Check sheet for the modelled part. Datum: model origin and axes. Units: mm. A direction names the side the tool comes from. Give positions to 0.01 mm unless a question says otherwise; leave off trailing zeros. Write each loop counter-clockwise with the first axis right and the second up, starting at its lowest first coordinate (ties: lowest second). Pieces come first, ordered by that corner, then holes. Notation, with made-up numbers: M -18,-14.5 L 28,-14.5 A24 cw 28,10.5 Z; hole C 57.5,57.5 d4. An arc over 180 degrees is marked long. Write item = value, one per line. Start each with the question number.
1) Sectioned sample at A-A, the plane y = -18.5. Record the cut outline in (x, z).
2) Set-up check for faces 1 (the face through (0, 23, 16)), 2 (the face through (23, 2.25, 24)), 3 (the face through (0, 21, 18)): record each of +Z, -Z, +X, -X, +Y, -Y from which the full face is reachable in a straight line by a thin tool's end or side.
3) Sectioned sample at C-C, the plane z = 18. Record the cut outline in (x, y), then the cut area to 3 significant figures.
4) Gauge pin test, flat ends, axial feed: pin 1 (1 mm diameter, centred on y = -1.5, z = 28, fed in from +X); pin 2 (1.5 mm diameter, centred on x = 3, y = -11, fed in from -Z); pin 3 (5 mm diameter, centred on x = 17.5, y = 5.5, fed in from +Z). Record the tip position at first contact, or that the pin passes through.
5) Scan lines: L1, parallel to X at y = -9, z = 21; L2, parallel to Y at x = 16, z = 11.5; L3, parallel to Z at x = -13.5, y = -9.5. Record each from-to range of solid material in increasing order.
6) Sectioned sample at B-B, the plane x = -17. Record the cut outline in (y, z).
7) Draft check along Y on faces 4 (the face through (0, -21, 18)), 5 (the face through (-23.75, 0, 16)), 6 (the face through (0, -23, 16)), 7 (the face through (-21.75, 0, 18)). Enter one of: pulls with the +Y half, pulls with the -Y half, needs draft (parallel to the pull), parting line crosses it, or undercut.
from build123d import *

# Parameters (mm, degrees)
F0_W     = 47.5
F0_H     = 46
F1_DEPTH = 33
F2_W     = 43.5
F2_H     = 42
F3_DEPTH = 31
F5_DEPTH = 5


with BuildPart() as f1:
    # F0 (on Top) → F1 (new body)
    with BuildSketch(Plane.XY):
        Rectangle(F0_W, F0_H)
    extrude(amount=F1_DEPTH)

    # F2 (on face) → F3 (cut)
    with BuildSketch(Plane.XY.offset(33)):
        Rectangle(F2_W, F2_H)
    extrude(amount=-F3_DEPTH, mode=Mode.SUBTRACT)

    # F4 (on face) → F5 (cut)
    with BuildSketch(Plane.YZ.offset(23.75)):
        with BuildLine():
            ThreePointArc((-2.25, 16.043559), (0, 18.293559), (2.25, 16.043559))
            Line((2.25, 16.043559), (2.25, 33))
            Line((2.25, 33), (-2.25, 33))
            Line((-2.25, 33), (-2.25, 16.043559))
        make_face()
        with BuildLine():
            ThreePointArc((-2.25, 16.043559), (0, 13.793559), (2.25, 16.043559))
            ThreePointArc((2.25, 16.043559), (0, 18.293559), (-2.25, 16.043559))
        make_face()
    extrude(amount=-F5_DEPTH, mode=Mode.SUBTRACT)


solid = f1.part
Data:
q1.outline = M -23.75,0 L 23.75,0 L 23.75,33 L 21.75,33 L 21.75,2 L -21.75,2 L -21.75,33 L -23.75,33 Z
q2.face_1 = +Z, -Z, +X, -X, +Y
q2.face_2 = +Z, +X
q2.face_3 = +Z
q3.outline = M -23.75,-23 L 23.75,-23 L 23.75,-2.25 L 21.75,-2.25 L 21.75,-21 L -21.75,-21 L -21.75,21 L 21.75,21 L 21.75,2.25 L 23.75,2.25 L 23.75,23 L -23.75,23 Z
q3.area = 349 mm2
q4.pin_1 = -21.75
q4.pin_2 = 0
q4.pin_3 = 2
q5.L1 = -23.75 to -21.75, 21.75 to 23.75
q5.L2 = -23 to -21, 21 to 23
q5.L3 = 0 to 2
q6.outline = M -23,0 L 23,0 L 23,33 L 21,33 L 21,2 L -21,2 L -21,33 L -23,33 Z
q7.face_4 = undercut
q7.face_5 = needs draft
q7.face_6 = pulls with the -Y half
q7.face_7 = undercut
